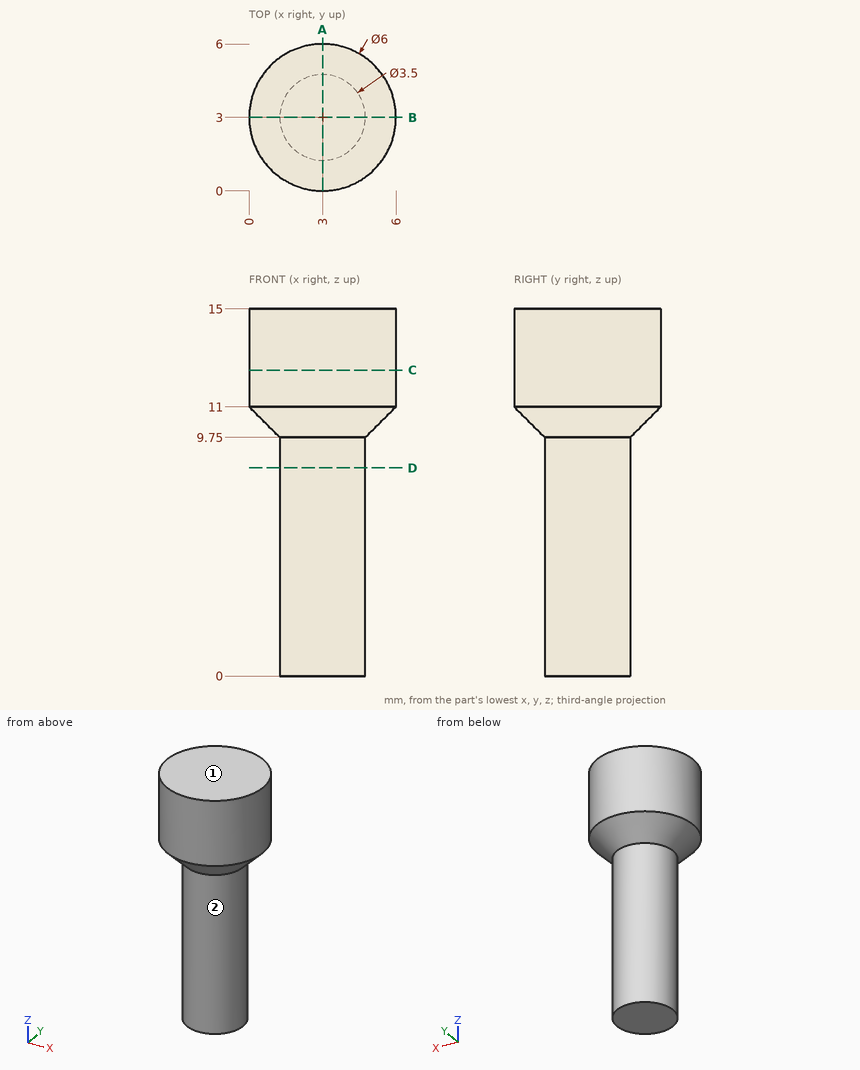
Job drawing, mm, ordinate dimensions from the low corner. One solid piece. Coordinates: 2 decimals unless noted, no trailing zeros. Order: outer loops, then holes, each group sorted by start corner. A loop starts at its lowest first (then second) coordinate and runs counter-clockwise, first axis right, second up. Notation, with made-up numbers: M 22.25,-4 L 79.25,-4 A32 cw 79.25,22 Z; hole C 16.5,57.5 d1. An arc over 180 degrees is marked long. Return JSON: item names as keys, results as strings.
1. Flat gauge pins, fed straight in: pin 1 (1.5 mm diameter, centred on x = 3.5, y = 3.5, fed in from -Z); pin 2 (2 mm diameter, centred on y = 5, z = 9.5, fed in from -X). Where does each tip first touch, or does it go through?
Ans:
{"pin 1": "z = 0", "pin 2": "x = 1.17"}
2. Saw through at A-A (x = 3). Give the cut face in (y, z), and give its area (3 significant figures).
Ans:
{"outline": "M 0,11 L 1.25,9.75 L 1.25,0 L 4.75,0 L 4.75,9.75 L 6,11 L 6,15 L 0,15 Z", "area": "64.1 mm^2"}
3. Drill centre lines: probe 1 along Y at (x, z) = (2.85, 12.75); probe 2 along Z at (x, y) = (3.3, 5.35); probe 3 along X at (y, z) = (4.3, 11.75). Where is each one in solid material? Low to high.
Ans:
{"probe 1": "0 to 6", "probe 2": "10.37 to 15", "probe 3": "0.3 to 5.7"}
4. Saw through at D-D (z = 8.5). Give the cut face in (x, y), and give its area (3 significant figures).
Ans:
{"outline": "C 3,3 d3.5", "area": "9.62 mm^2"}
5. Pull direction X, two halves, no side cores. Call the marked faces 1 and 2: +X half, -X half, draft (parallel to the pull), parting line (faces both ways), or undercut.
Ans:
{"face 1": "draft", "face 2": "parting line"}
6. Saw through at C-C (z = 12.5). Give the cut face in (x, y), and give its area (3 significant figures).
Ans:
{"outline": "C 3,3 d6", "area": "28.3 mm^2"}
